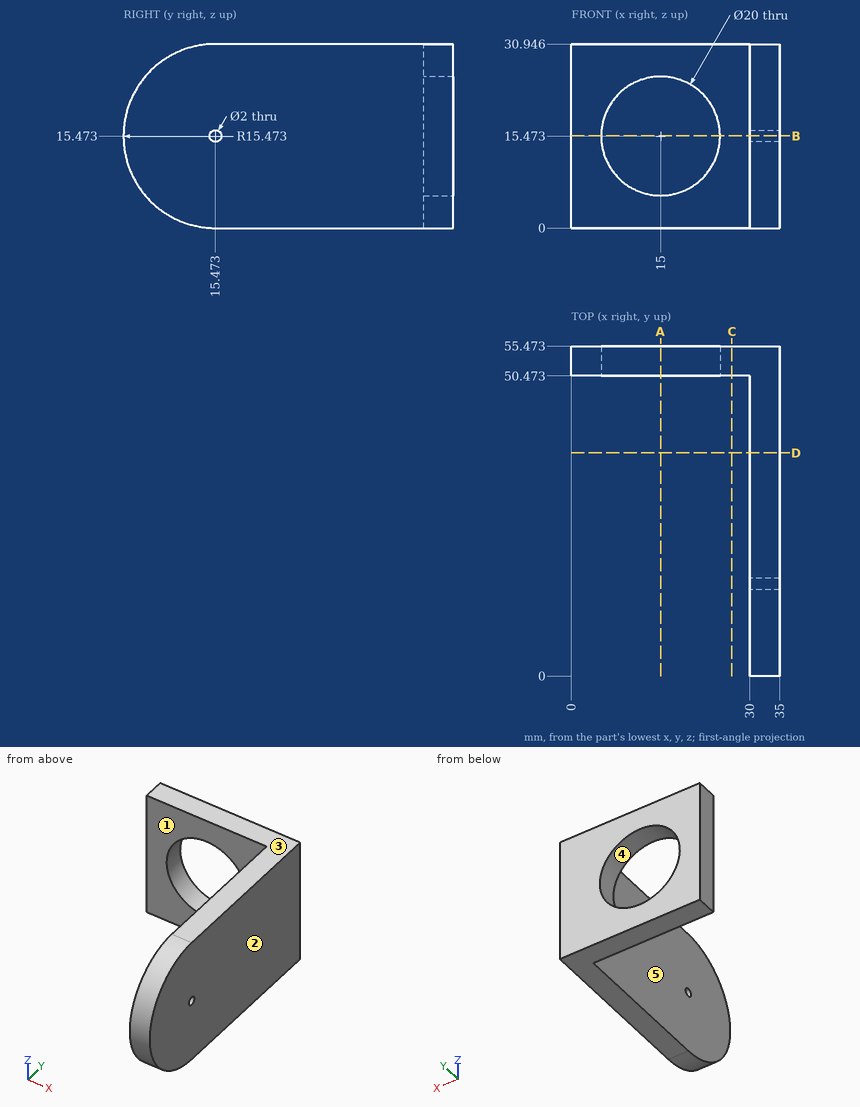
Design review of the part shown in the three views and the two pictorial views. Dimensions are in mm from the part's minimum x, y and z. A direction names the side the tool comes from. Give positions to 0.01 mm unless a question says otherwise; leave off trailing zeros. Loops run counter-clockwise (first coordinate to the right, second up) from the corner with the lowest first, then second, coordinate; pieces in that order, holes last. Notation, with made-up numbers: (1.5, -6) - (44.5, -6) arc R25 ccw to (44.5, 19) - close; hole circle Ø11 at (22, -27). An arc over 180 degrees is marked (long way). Use CSV: the item, a comma, the result in double quotes. Start each with the question number.
1. Add section C-C (x = 27). State the section outline as (y, z) points.
2. Add section A-A (x = 15). State the section outline as (y, z) points, plus the area to 3 significant figures.
3. Draft analysis for pull direction X (two halves, no side actions). For the marked faces 3, 4 and 5, state which applies: released by +X, released by -X, zero draft, split by the parting line, or undercut.
4. Machinability: for the marked faces 1 and 2, which of the approach directions +Z, -Z, +X, -X, +Y, -Y give a long, thin tool a straight path to every point of the face, cutting with its end or side? Answer none if there is none.
5. Insertion check: P1, Ø3, axis at y = 15.47, z = 15.47, coming from the -X side; P2, Ø8, axis at x = 8.5, z = 25.5, coming from the -Y side. Each pin has a flat end and moves straight along its axis. Give the tip position at first contact, or say it passes through.
6. Add section B-B (z = 15.5). State the section outline as (x, y) points.
7. Wall thickness on L1, parallel to Y at x = 10.5, z = 25; L2, parallel to X at y = 7.5, z = 18; L3, parallel to X at y = 51.5, z = 9: over which ranges is each line inside the solid? List them lowest first.
8. Add section D-D (y = 37.5). State the section outline as (x, z) points, plus the area to 3 significant figures.
Results found:
1,outline,"(50.47, 0) - (55.47, 0) - (55.47, 30.95) - (50.47, 30.95) - close"
2,outline,"(50.47, 0) - (55.47, 0) - (55.47, 5.47) - (50.47, 5.47) - close; (50.47, 25.47) - (55.47, 25.47) - (55.47, 30.95) - (50.47, 30.95) - close"
2,area,"54.7 mm²"
3,face 3,"zero draft"
3,face 4,"undercut"
3,face 5,"released by -X"
4,face 1,"+Z, -Z, -X, -Y"
4,face 2,"+Z, -Z, +X, +Y, -Y"
5,P1,"stops at x = 30"
5,P2,"stops at y = 50.47"
6,outline,"(0, 50.47) - (5, 50.47) - (5, 55.47) - (0, 55.47) - close; (25, 50.47) - (30, 50.47) - (30, 16.47) - (35, 16.47) - (35, 55.47) - (25, 55.47) - close; (30, 0) - (35, 0) - (35, 14.47) - (30, 14.47) - close"
7,L1,"y = 50.47 to 55.47"
7,L2,"x = 30 to 35"
7,L3,"x = 0 to 7.38, 22.62 to 35"
8,outline,"(30, 0) - (35, 0) - (35, 30.95) - (30, 30.95) - close"
8,area,"155 mm²"
